Geometry: final body of the model. Coordinates: model frame, mm. Give positions to 0.01 mm unless a question says otherwise; leave off trailing zeros. Write each loop counter-clockwise with the first axis right and the second up, starting at its lowest first coordinate (ties: lowest second). Pieces come first, ordered by that corner, then holes.
Q1. Pin query (flat end, axial travel): pin 1 Ø3 at (x, z) = (6.74, 6.74) entering from +Y; pin 2 Ø10 at (x, z) = (-36, 60) entering from -Y; pin 3 Ø1.5 at (y, z) = (1.5, -73) entering from +X. Return the tip coordinate at first contact, or that it passes through.
Q2. Section C-C (x = 90). Return the cut outline in (y, z) (3 decimals), plus the area to 3 significant figures.
Q3. Section B-B (z = -69). Return the cut outline in (x, y) (3 decimals).
Q4. Line query: line 1 (Z direction, x = 0, y = 0.85) (3 decimals); line 2 (Z direction, x = 42, y = 2); line 3 (X direction, y = 0.8, z = -74). Output: solid intervals per line, ascending.
Q5. Section A-A (y = 1.3). State how many separate pieces and enclosed holes the cut face has, plus the area to 3 significant figures.
from build123d import *

# Parameters (mm, degrees)
SKETCH1_R           = 152.4
BOSS_EXTRUDE1_DEPTH = 3.175
CUT_EXTRUDE1_REACH  = 5.175
SKETCH2_R           = 3.175
SKETCH2_R_2         = 1.5875


with BuildPart() as part:
    # Sketch1 → Boss-Extrude1 (new body)
    with BuildSketch(Plane(origin=(0, 0, 0), x_dir=(1, 0, 0), z_dir=(0, 1, 0))):
        Circle(SKETCH1_R)
    extrude(amount=BOSS_EXTRUDE1_DEPTH)

    # Sketch2 → Cut-Extrude1 (cut, up to next)
    with BuildSketch(Plane(origin=(0, 3.175, 0), x_dir=(1, 0, 0), z_dir=(0, 1, 0)), mode=Mode.PRIVATE) as cut_extrude1_sk1:
        Circle(SKETCH2_R)
    cut_extrude1_tool1 = extrude(cut_extrude1_sk1.sketch, amount=-CUT_EXTRUDE1_REACH, mode=Mode.PRIVATE) & part.part
    add(cut_extrude1_tool1.solids().sort_by_distance((0, 3.175, 0))[0], mode=Mode.SUBTRACT)
    # Sketch2 → Cut-Extrude1 (cut, up to next)
    with BuildSketch(Plane(origin=(0, 3.175, 0), x_dir=(1, 0, 0), z_dir=(0, 1, 0)), mode=Mode.PRIVATE) as cut_extrude1_sk2:
        with Locations((6.735192091, 6.735192091)):
            Circle(SKETCH2_R_2)
    cut_extrude1_tool2 = extrude(cut_extrude1_sk2.sketch, amount=-CUT_EXTRUDE1_REACH, mode=Mode.PRIVATE) & part.part
    add(cut_extrude1_tool2.solids().sort_by_distance((6.735192, 3.175, -6.735192))[0], mode=Mode.SUBTRACT)
    # Sketch2 → Cut-Extrude1 (cut, up to next)
    with BuildSketch(Plane(origin=(0, 3.175, 0), x_dir=(1, 0, 0), z_dir=(0, 1, 0)), mode=Mode.PRIVATE) as cut_extrude1_sk3:
        with Locations((-6.735192091, 6.735192091)):
            Circle(SKETCH2_R_2)
    cut_extrude1_tool3 = extrude(cut_extrude1_sk3.sketch, amount=-CUT_EXTRUDE1_REACH, mode=Mode.PRIVATE) & part.part
    add(cut_extrude1_tool3.solids().sort_by_distance((-6.735192, 3.175, -6.735192))[0], mode=Mode.SUBTRACT)
    # Sketch2 → Cut-Extrude1 (cut, up to next)
    with BuildSketch(Plane(origin=(0, 3.175, 0), x_dir=(1, 0, 0), z_dir=(0, 1, 0)), mode=Mode.PRIVATE) as cut_extrude1_sk4:
        with Locations((-6.240150163, -7.19625951)):
            Circle(SKETCH2_R_2)
    cut_extrude1_tool4 = extrude(cut_extrude1_sk4.sketch, amount=-CUT_EXTRUDE1_REACH, mode=Mode.PRIVATE) & part.part
    add(cut_extrude1_tool4.solids().sort_by_distance((-6.24015, 3.175, 7.19626))[0], mode=Mode.SUBTRACT)
    # Sketch2 → Cut-Extrude1 (cut, up to next)
    with BuildSketch(Plane(origin=(0, 3.175, 0), x_dir=(1, 0, 0), z_dir=(0, 1, 0)), mode=Mode.PRIVATE) as cut_extrude1_sk5:
        with Locations((6.735192091, -6.735192091)):
            Circle(SKETCH2_R_2)
    cut_extrude1_tool5 = extrude(cut_extrude1_sk5.sketch, amount=-CUT_EXTRUDE1_REACH, mode=Mode.PRIVATE) & part.part
    add(cut_extrude1_tool5.solids().sort_by_distance((6.735192, 3.175, 6.735192))[0], mode=Mode.SUBTRACT)


solid = part.part
Computed:
1. pin 1: passes through
1. pin 2: stops at y = 0
1. pin 3: stops at x = 134.19
2. outline: (0, -122.987) - (3.175, -122.987) - (3.175, 122.987) - (0, 122.987) - close
2. area: 781 mm2
3. outline: (-135.885, 0) - (135.885, 0) - (135.885, 3.175) - (-135.885, 3.175) - close
4. line 1: z = -152.4 to -3.175, 3.175 to 152.4
4. line 2: z = -146.5 to 146.5
4. line 3: x = -133.23 to 133.23
5. separate pieces: 1
5. enclosed holes: 5
5. area: 72,900 mm2
